Autodesk Inventor part; units mm, degrees
ref_plane "YZ Plane" through (0, 0, 0) normal (1, 0, 0) x (0, 1, 0)
ref_plane "XZ Plane" through (0, 0, 0) normal (0, 1, 0) x (-1, 0, 0)
ref_plane "XY Plane" through (0, 0, 0) normal (0, 0, 1) x (1, 0, 0)
sketch "Sketch1" plane through (0, 0, 0) normal (0, 0, 1) x (1, 0, 0)
  line L0 (10, -10.0138) -> (-10, -10.0138)
  line L1 (-10, -10.0138) -> (-10, 10.0138)
  line L2 (-10, 10.0138) -> (10, 10.0138)
  line L3 (10, 10.0138) -> (10, -10.0138)
  line L4 (10, -10.0138) -> (-10, 10.0138) construction
  line L5 (-10, -10.0138) -> (10, 10.0138) construction
  point P0 (0, 0)
  dimension "d0" = 20
extrude "Extrusion1" add sketch "Sketch1" along normal mid plane 20
sketch "Sketch2" plane through (0, 0, 10) normal (0, 0, 1) x (1, 0, 0)
  line L0 (10, 10.0138) -> (-10, 10.0138)
  line L1 (-10, 10.0138) -> (-10, -10.0138)
  line L2 (-10, -10.0138) -> (10, -10.0138)
  line L3 (10, -10.0138) -> (10, 10.0138)
  point P0 (0, 0)
sketch "Sketch3" plane through (-10, 10.0138, 10) normal (0, 1, 0) x (1, 0, 0)
  line L0 (10, 10) -> (3.9087, 16.7786)
  line L1 (3.9087, 16.7786) -> (6.1897, 16.7786)
  line L2 (6.1897, 16.7786) -> (11.262, 11.134)
  line L3 (11.262, 11.134) -> (16.1719, 5.6701)
  line L4 (16.1719, 5.6701) -> (13.8909, 5.6701)
  line L5 (13.8909, 5.6701) -> (10, 10)
  line L6 (11.262, 11.134) -> (16.1719, 16.7786)
  line L7 (16.1719, 16.7786) -> (13.8909, 16.7786)
  line L8 (13.8909, 16.7786) -> (10.1029, 12.4238)
  line L9 (3.9087, 5.6701) -> (8.981, 11.134)
  line L10 (10.1029, 9.8855) -> (6.1897, 5.6701)
  line L11 (6.1897, 5.6701) -> (3.9087, 5.6701)
extrude "Extrusion2" cut sketch "Sketch3" against normal blind 1
sketch "Sketch4" plane through (0, 0, -10) normal (0, 0, -1) x (-1, 0, 0)
  line L0 (6.35, -6.35) -> (-6.35, -6.35)
  line L1 (-6.35, -6.35) -> (6.35, 6.35)
  line L2 (6.35, 6.35) -> (-6.35, 6.35)
  line L3 (6.35, -6.35) -> (6.35, -4.7625)
  line L4 (6.35, -4.7625) -> (-3.175, -4.7625)
  line L5 (-3.175, -4.7625) -> (6.35, 4.7625)
  line L6 (6.35, 4.7625) -> (-6.35, 4.7625)
  line L7 (6.35, 4.7625) -> (6.35, 6.35)
  line L8 (-6.35, 4.7625) -> (-6.35, 6.35)
  line L9 (-4.7625, -6.35) -> (-3.175, -4.7625)
  point P0 (0, 0)
  point P1 (4.7625, 4.7625)
extrude "Extrusion3" cut sketch "Sketch4" against normal blind 1
sketch "Sketch5" plane through (10, -10.0138, 10) normal (1, 0, 0) x (0, 0, -1)
  line L0 (5.3355, 9.1946) -> (5.3355, 10.8331)
  line L1 (5.3355, 10.8331) -> (10.3819, 10.8331)
  line L2 (10.3897, 9.1946) -> (5.3355, 9.1946)
  line L3 (10.3819, 10.8331) -> (15.9139, 14.2248)
  line L4 (15.9139, 14.2248) -> (16.6235, 13.0674)
  line L5 (16.6235, 13.0674) -> (11.6534, 10.0201)
  line L6 (11.6534, 10.0201) -> (16.5746, 7.0635)
  line L7 (16.5746, 7.0635) -> (15.875, 5.899)
  line L8 (15.875, 5.899) -> (10.3897, 9.1946)
  point P0 (10, 10.0138)
  point P1 (5.3355, 10.0138)
extrude "Extrusion4" cut sketch "Sketch5" against normal blind 1
equation "\"d1\" = d0"
properties part number "Cubo-001-001_3DPrint"
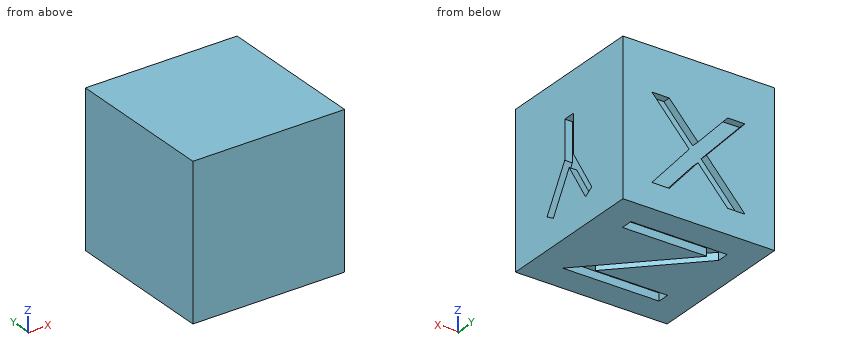
CAD build for the part. Positions are in the model's coordinates, mm. Round coordinates to 2 decimals unless told otherwise and drop trailing zeros. Order: outer loops, then holes, each group sorted by start corner. A loop starts at its lowest first (then second) coordinate and runs counter-clockwise, first axis right, second up. Notation, with made-up numbers: (-13, 3) -> (38, 3) arc R32 ccw to (38, 29) -> close; hole circle Ø9 at (-7.5, 9.5). An arc over 180 degrees is marked (long way). Write each question's results on one line, items separated by ' | '.
1. Cut at B-B (x = -1.75). Give the cut face in (y, z).
Findings below:
outline: (-10.01, -10) -> (-6.35, -10) -> (-6.35, -9) -> (-4.76, -9) -> (-4.76, -10) -> (0.16, -10) -> (0.16, -9) -> (1.75, -9) -> (1.75, -10) -> (4.76, -10) -> (4.76, -9) -> (6.35, -9) -> (6.35, -10) -> (10.01, -10) -> (10.01, -4.49) -> (9.01, -4.49) -> (9.01, -1.95) -> (10.01, -1.95) -> (10.01, -0.35) -> (9.01, -0.35) -> (9.01, 2.11) -> (10.01, 2.11) -> (10.01, 10) -> (-10.01, 10) -> close
2. Cut at D-D (z = -4.75). Give the cut face in (x, y).
Findings below:
outline: (-10, -10.01) -> (10, -10.01) -> (10, -3.44) -> (9, -3.44) -> (9, -1.85) -> (10, -1.85) -> (10, 1.9) -> (9, 1.9) -> (9, 3.5) -> (10, 3.5) -> (10, 10.01) -> (4.41, 10.01) -> (4.41, 9.01) -> (2.13, 9.01) -> (2.13, 10.01) -> (-1.99, 10.01) -> (-1.99, 9.01) -> (-4.27, 9.01) -> (-4.27, 10.01) -> (-10, 10.01) -> close
3. Cut at C-C (z = 1.75). Give the cut face in (x, y), plus the area to 3 significant figures.
Findings below:
outline: (-10, -10.01) -> (10, -10.01) -> (10, -0.82) -> (9, -0.82) -> (9, 0.82) -> (10, 0.82) -> (10, 10.01) -> (3.85, 10.01) -> (3.85, 9.01) -> (1.57, 9.01) -> (1.57, 10.01) -> (-1.42, 10.01) -> (-1.42, 9.01) -> (-3.7, 9.01) -> (-3.7, 10.01) -> (-10, 10.01) -> close | area: 394 mm²
4. Wall check: line 1 along X through (y, z) = (-0.5, -1.25); line 2 along Z through (x, y) = (2, 6). Give the ranges that are in metal, low to high. Write a range as [from, to].
Findings below:
line 1: x = [-10, 9] | line 2: z = [-9, 10]
5. Cut at A-A (y = -6). Give the cut face in (x, z).
Findings below:
outline: (-10, -10) -> (-6.35, -10) -> (-6.35, -9) -> (6, -9) -> (6, -10) -> (10, -10) -> (10, 10) -> (-10, 10) -> close
